Verification items for the finished model (mm, model axes). A direction names the side the tool comes from. Round coordinates to 2 decimals unless told otherwise and drop trailing zeros. Write each loop counter-clockwise with the first axis right and the second up, starting at its lowest first coordinate (ties: lowest second). Pieces come first, ordered by that corner, then holes. Notation, with made-up numbers: (55.5, 81) - (99.5, 81) arc R17 ccw to (99.5, 104) - close; hole circle Ø7 at (11.25, 37). An arc over 180 degrees is marked (long way). Answer as a JSON object with one key per item and string values.
```python
from build123d import *

# Parameters (mm, degrees)
F1_DEPTH = 3
F2_R     = 2
F3_DEPTH = 40


with BuildPart() as f1:
    # F0 (on Top) → F1 (new body)
    with BuildSketch(Plane.XY):
        with BuildLine():
            Line((11.7317076979, 4.315632835), (-8.2682923021, 4.315632835))
            Line((-8.2682923021, 4.315632835), (-8.2682923021, 0.315632835))
            Line((-8.2682923021, 0.315632835), (-1.7682923021, 0.315632835))
            ThreePointArc((-1.7682923021, 0.315632835), (-0.2682923021, 1.815632835), (1.2317076979, 0.315632835))
            Line((1.2317076979, 0.315632835), (11.7317076979, 0.315632835))
            Line((11.7317076979, 0.315632835), (11.7317076979, 4.315632835))
        make_face()
        with BuildLine():
            Line((31.7317076979, 4.315632835), (11.7317076979, 4.315632835))
            Line((11.7317076979, 4.315632835), (11.7317076979, 0.315632835))
            Line((11.7317076979, 0.315632835), (22.2317076979, 0.315632835))
            ThreePointArc((22.2317076979, 0.315632835), (23.7317076979, 1.815632835), (25.2317076979, 0.315632835))
            Line((25.2317076979, 0.315632835), (31.7317076979, 0.315632835))
            Line((31.7317076979, 0.315632835), (31.7317076979, 4.315632835))
        make_face()
        with BuildLine():
            Line((-1.7682923021, 0.315632835), (-8.2682923021, 0.315632835))
            Line((-8.2682923021, 0.315632835), (-8.2682923021, -3.684367165))
            Line((-8.2682923021, -3.684367165), (11.7317076979, -3.684367165))
            Line((11.7317076979, -3.684367165), (11.7317076979, 0.315632835))
            Line((11.7317076979, 0.315632835), (1.2317076979, 0.315632835))
            ThreePointArc((1.2317076979, 0.315632835), (-0.2682923021, -1.184367165), (-1.7682923021, 0.315632835))
        make_face()
        with BuildLine():
            Line((22.2317076979, 0.315632835), (11.7317076979, 0.315632835))
            Line((11.7317076979, 0.315632835), (11.7317076979, -3.684367165))
            Line((11.7317076979, -3.684367165), (31.7317076979, -3.684367165))
            Line((31.7317076979, -3.684367165), (31.7317076979, 0.315632835))
            Line((31.7317076979, 0.315632835), (25.2317076979, 0.315632835))
            ThreePointArc((25.2317076979, 0.315632835), (23.7317076979, -1.184367165), (22.2317076979, 0.315632835))
        make_face()
        with BuildLine():
            Line((1.2317076979, 0.315632835), (-1.7682923021, 0.315632835))
            ThreePointArc((-1.7682923021, 0.315632835), (-0.2682923021, -1.184367165), (1.2317076979, 0.315632835))
        make_face()
        with BuildLine():
            ThreePointArc((1.2317076979, 0.315632835), (-0.2682923021, 1.815632835), (-1.7682923021, 0.315632835))
            Line((-1.7682923021, 0.315632835), (1.2317076979, 0.315632835))
        make_face()
        with BuildLine():
            ThreePointArc((25.2317076979, 0.315632835), (23.7317076979, 1.815632835), (22.2317076979, 0.315632835))
            Line((22.2317076979, 0.315632835), (25.2317076979, 0.315632835))
        make_face()
        with BuildLine():
            Line((25.2317076979, 0.315632835), (22.2317076979, 0.315632835))
            ThreePointArc((22.2317076979, 0.315632835), (23.7317076979, -1.184367165), (25.2317076979, 0.315632835))
        make_face()
    extrude(amount=-F1_DEPTH)

    # F2
    f2_edges = [f1.edges().sort_by_distance(p)[0] for p in [
        (-8.268292, -3.684367, -1.5),
        (-8.268292, 4.315633, -1.5),
        (31.731708, -3.684367, -1.5),
        (31.731708, 4.315633, -1.5),
    ]]
    fillet(f2_edges, radius=F2_R)

    # F0 (on Top) → F3 (join)
    with BuildSketch(Plane.XY):
        with BuildLine():
            ThreePointArc((1.2317076979, 0.315632835), (-0.2682923021, 1.815632835), (-1.7682923021, 0.315632835))
            Line((-1.7682923021, 0.315632835), (1.2317076979, 0.315632835))
        make_face()
        with BuildLine():
            Line((1.2317076979, 0.315632835), (-1.7682923021, 0.315632835))
            ThreePointArc((-1.7682923021, 0.315632835), (-0.2682923021, -1.184367165), (1.2317076979, 0.315632835))
        make_face()
        with BuildLine():
            ThreePointArc((25.2317076979, 0.315632835), (23.7317076979, 1.815632835), (22.2317076979, 0.315632835))
            Line((22.2317076979, 0.315632835), (25.2317076979, 0.315632835))
        make_face()
        with BuildLine():
            Line((25.2317076979, 0.315632835), (22.2317076979, 0.315632835))
            ThreePointArc((22.2317076979, 0.315632835), (23.7317076979, -1.184367165), (25.2317076979, 0.315632835))
        make_face()
    extrude(amount=F3_DEPTH)


solid = f1.part
```
Q1. Set-up check for faces 5 (the flat face through (11, -3.684, -1)), 6 (the cylindrical face through (1.23, 0.25, 19.72)): record each of +Z, -Z, +X, -X, +Y, -Y from which the full face is reachable in a straight line by a thin tool's end or side.
Geometry check:
{"face 5": "+Z, -Z, +X, -X, -Y", "face 6": "+Z"}
Q2. Section check B-B, the plane x = 16.5. Record the cut outline in (y, z).
Geometry check:
{"outline": "(-3.68, -3) - (4.32, -3) - (4.32, 0) - (-3.68, 0) - close"}
Q3. Material ranges on line 1 along Z through (x, y) = (5.5, 3.5); line 2 along X through (y, z) = (0.75, 18.5); line 3 along X through (y, z) = (1.25, 20), recorded low to high. Write a range as [from, to].
Geometry check:
{"line 1": "z = [-3, 0]", "line 2": "x = [-1.7, 1.17], [22.3, 25.17]", "line 3": "x = [-1.44, 0.91], [22.56, 24.91]"}
Q4. Gauge pin test, flat ends, axial feed: P1, Ø2.5, axis at x = 16, y = 0, coming from the +Z side; P2, Ø6, axis at x = 2.5, z = 12, coming from the -Y side. Record the tip position at first contact, or that the pin passes through.
Geometry check:
{"P1": "stops at z = 0", "P2": "stops at y = -1.18"}
Q5. Section check C-C, the plane y = -2.25. Record the cut outline in (x, z), then the cut area to 3 significant figures.
Geometry check:
{"outline": "(-8.19, -3) - (31.65, -3) - (31.65, 0) - (-8.19, 0) - close", "area": "120 mm2"}
Q6. Section check A-A, the plane z = 17. Record the cut outline in (x, y), then the cut area to 3 significant figures.
Geometry check:
{"outline": "circle Ø3 at (-0.27, 0.32); circle Ø3 at (23.73, 0.32)", "area": "14.1 mm2"}
Q7. Release check for a two-part mould opening along X. For faces 1 (the flat face through (11, 0, 0)), 2 (the flat face through (0, 0, 40)), 3 (the flat face through (-8.268, 0, -1)), 4 (the cylindrical face through (22.3, -0.13, 19.72)) record: released by +X, released by -X, zero draft, split by the parting line, or undercut.
Geometry check:
{"face 1": "undercut", "face 2": "zero draft", "face 3": "released by -X", "face 4": "undercut"}
